from build123d import *

# Parameters (mm, degrees)
SKETCH1_W             = 228.6
SKETCH1_H             = 254
BOSS_EXTRUDE1_DEPTH   = 6.35
F_4_40_TAPPED_HOLE1_D = 2.2606
F_4_40_TAPPED_HOLE2_D = 2.2606


with BuildPart() as part:
    # Sketch1 → Boss-Extrude1 (new body)
    with BuildSketch(Plane(origin=(0, 0, 0), x_dir=(1, 0, 0), z_dir=(0, 1, 0))):
        with Locations((114.3, 127)):
            Rectangle(SKETCH1_W, SKETCH1_H)
    extrude(amount=BOSS_EXTRUDE1_DEPTH)

    # #4-40 Tapped Hole1 (through all)
    with Locations(Plane(origin=(0, 6.35, 0), x_dir=(1, 0, 0), z_dir=(0, 1, 0))):
        with Locations((15.735159407, 43.18), (15.875, 58.42), (84.05884141, 57.388437181), (144.561688198, 57.388437181), (0, 127), (144.561688198, 196.611562819), (84.05884141, 196.611562819), (15.875, 195.58), (15.735159407, 210.82), (114.3, 0), (212.864840593, 43.18), (212.725, 58.42), (212.864840593, 210.82), (212.725, 195.58), (228.6, 127), (114.3, 254)):
            Hole(F_4_40_TAPPED_HOLE1_D / 2)

    # #4-40 Tapped Hole2 (through all)
    with Locations(Plane(origin=(0, 6.35, 0), x_dir=(1, 0, 0), z_dir=(0, 1, 0))):
        with Locations((58.65884141, 59.18949303), (58.65884141, 42.0497), (169.961688198, 59.18949303), (169.961688198, 42.0497)):
            Hole(F_4_40_TAPPED_HOLE2_D / 2)


solid = part.part
The listing builds one solid part. Answer for the finished solid, in the listing's coordinates (mm). Round coordinates to 2 decimals unless told otherwise and drop trailing zeros. Answer in a Markdown table with one row per item. Add a question column.
1) Determine the mould class of faces 1 (the face through (171, 3, 0)), 2 (the face through (0, 3, -190)), 3 (the face through (56, 3, -254)) for opening direction Z: pulls with the +Z half, pulls with the -Z half, needs draft (parallel to the pull), parting line crosses it, or undercut.
2) Consider line 1 along X through (y, z) = (2.25, -210.82); line 2 along X through (y, z) = (3.25, -195.58). Determine where each line is inside the solid, lowest interval first. Write a range as from..to.
3) A flat-ended cylindrical pin translates along its axis: pin 1 Ø1.8 at (x, z) = (58.66, -59.19) entering from -Y. Find the tip coordinate at first contact, or state that the pin passes through.
Findings below:
| question | item | result |
|---|---|---|
| 1 | face 1 | pulls with the +Z half |
| 1 | face 2 | needs draft |
| 1 | face 3 | pulls with the -Z half |
| 2 | line 1 | x = 0..14.6, 16.87..211.73, 214..228.6 |
| 2 | line 2 | x = 0..14.74, 17.01..83.6, 84.52..144.1, 145.02..211.59, 213.86..228.6 |
| 3 | pin 1 | passes through |
